Autodesk Inventor part; units mm, degrees
ref_plane "YZ Plane" through (0, 0, 0) normal (1, 0, 0) x (0, 1, 0)
ref_plane "XZ Plane" through (0, 0, 0) normal (0, 1, 0) x (-1, 0, 0)
ref_plane "XY Plane" through (0, 0, 0) normal (0, 0, 1) x (1, 0, 0)
sketch "Sketch1" plane through (0, 0, 0) normal (0, 0, 1) x (1, 0, 0)
  line L0 (0, 0) -> (32, 0)
  line L1 (32, 0) -> (32, 10)
  line L2 (32, 10) -> (0, 10)
  line L3 (0, 10) -> (0, 0)
  dimension "d0" = 32
  dimension "d1" = 10
extrude "Extrusion1" add sketch "Sketch1" along normal blind 2
sketch "Sketch2" plane through (0, 0, 2) normal (0, 0, 1) x (1, 0, 0)
  line L0 (32, 10) -> (0, 10)
  line L1 (0, 10) -> (0, 0)
  circle A0 centre (16, 5) radius 1.5
  point P0 (16, 10)
  point P1 (0, 5)
  dimension "d4" = 3
extrude "Extrusion2" cut sketch "Sketch2" against normal through all
sketch "Sketch3" plane through (32, 0, 0) normal (1, 0, 0) x (0, 0, -1)
  circle A0 centre (-10, 13.2398) radius 5 construction
  line L0 (0, 0) -> (0, 10)
  line L1 (-2, 10) -> (-2, 0)
  line L2 (-2, 0) -> (-13.2139, 9.4096)
  line L3 (0, 10) -> (-6.3819, 16.6909)
  arc A1 (-6.3819, 16.6909) -> (-13.2139, 9.4096) centre (-10, 13.2398) ccw
  circle A2 centre (-10, 13.2398) radius 1.5
  line L4 (0, 10) -> (-2, 10)
  dimension "d7" = 10
  dimension "d8" = 10
  dimension "d9" = 50
  dimension "d10" = 3
extrude "Extrusion3" add sketch "Sketch3" against normal blind 2
sketch "Sketch4" plane through (0, 0, 0) normal (-1, 0, 0) x (0, 0, 1)
  circle A0 centre (10, 13.2398) radius 1.5
  line L0 (6.3819, 16.6909) -> (0, 10)
  line L1 (2, 10) -> (0, 10)
  line L2 (2, 0) -> (2, 10)
  line L3 (2, 0) -> (13.2139, 9.4096)
  arc A1 (13.2139, 9.4096) -> (6.3819, 16.6909) centre (10, 13.2398) ccw
  point P0 (0, 0)
extrude "Extrusion4" add sketch "Sketch4" against normal blind 2
properties part number "Neck" material "ABS Plastic"
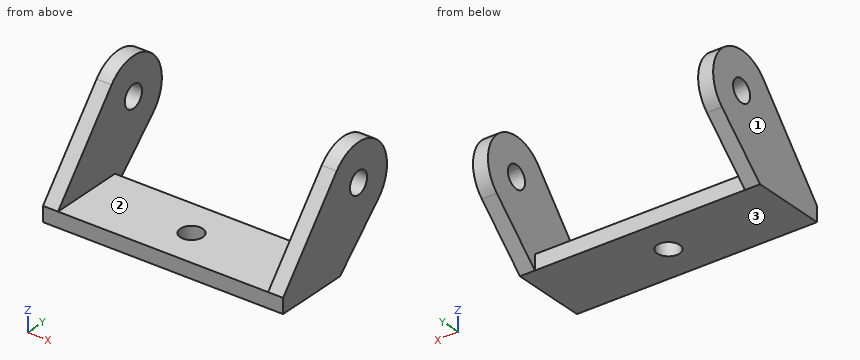
Work out the finished part from the listing and answer in its coordinate system (mm). Face numbers are marked on the shaded views. Give positions to 0.01 mm unless a question says otherwise; leave off trailing zeros. Order: outer loops, then holes, each group sorted by start corner. A loop starts at its lowest first (then second) coordinate and runs counter-clockwise, first axis right, second up. Notation, with made-up numbers: (-31.75, 79.25) -> (-14.75, 79.25) arc R17 ccw to (-14.75, 93.25) -> close; hole circle Ø9 at (-30.75, -17). An arc over 180 degrees is marked (long way). Answer as a JSON object with one key per item and string values. Group by question number.
1. The mould has two halves that part along X. Classify the marked faces 1, 2 and 3: released by +X, released by -X, zero draft, split by the parting line, or undercut.
2. Flat-ended cylindrical pins translate along their axes: pin 1 Ø8 at (x, y) = (18.5, 7) entering from +Z; pin 2 Ø1 at (x, z) = (9, 1) entering from +Y; pin 3 Ø4 at (x, z) = (28.5, 7) entering from +Y. Find the tip coordinate at first contact, or state that the pin passes through.
3. Consider line 1 along Y through (x, z) = (16, 1.5); line 2 along X through (y, z) = (14.5, 4.5); line 3 along Y through (x, z) = (5.5, 1). Determine where each line is inside the solid, lowest interval first. Write a range as [from, to].
4. Section D-D on y = 12.25 is taken. Determine the outline of the cut face in (x, z).
5. Section A-A on x = 16 is taken. Determine the outline of the cut face in (y, z), plus the area to 3 significant figures.
6. Section B-B on y = 4.25 is taken. Determine the outline of the cut face in (x, z).
7. Section C-C on z = 10 is taken. Determine the outline of the cut face in (x, y).
Result sheet:
{
 "1": {"face 1": "released by -X", "face 2": "undercut", "face 3": "zero draft"},
 "2": {"pin 1": "stops at z = 2", "pin 2": "stops at y = 10", "pin 3": "stops at y = 17.95"},
 "3": {"line 1": "y = [0, 3.5], [6.5, 10]", "line 2": "x = [0, 2], [30, 32]", "line 3": "y = [0, 10]"},
 "4": {"outline": "(0, 2.15) -> (2, 2.15) -> (2, 8.87) -> (0, 8.87) -> close; (0, 11.13) -> (2, 11.13) -> (2, 14.9) -> (0, 14.9) -> close; (30, 2.15) -> (32, 2.15) -> (32, 8.87) -> (30, 8.87) -> close; (30, 11.13) -> (32, 11.13) -> (32, 14.9) -> (30, 14.9) -> close"},
 "5": {"outline": "(0, 0) -> (3.5, 0) -> (3.5, 2) -> (0, 2) -> close; (6.5, 0) -> (10, 0) -> (10, 2) -> (6.5, 2) -> close", "area": "14.0 mm^2"},
 "6": {"outline": "(0, 0) -> (14.7, 0) -> (14.7, 2) -> (2, 2) -> (2, 7.06) -> (0, 7.06) -> close; (17.3, 0) -> (32, 0) -> (32, 7.06) -> (30, 7.06) -> (30, 2) -> (17.3, 2) -> close"},
 "7": {"outline": "(0, 6.71) -> (2, 6.71) -> (2, 11.74) -> (0, 11.74) -> close; (0, 14.74) -> (2, 14.74) -> (2, 18.24) -> (0, 18.24) -> close; (30, 6.71) -> (32, 6.71) -> (32, 11.74) -> (30, 11.74) -> close; (30, 14.74) -> (32, 14.74) -> (32, 18.24) -> (30, 18.24) -> close"}
}
